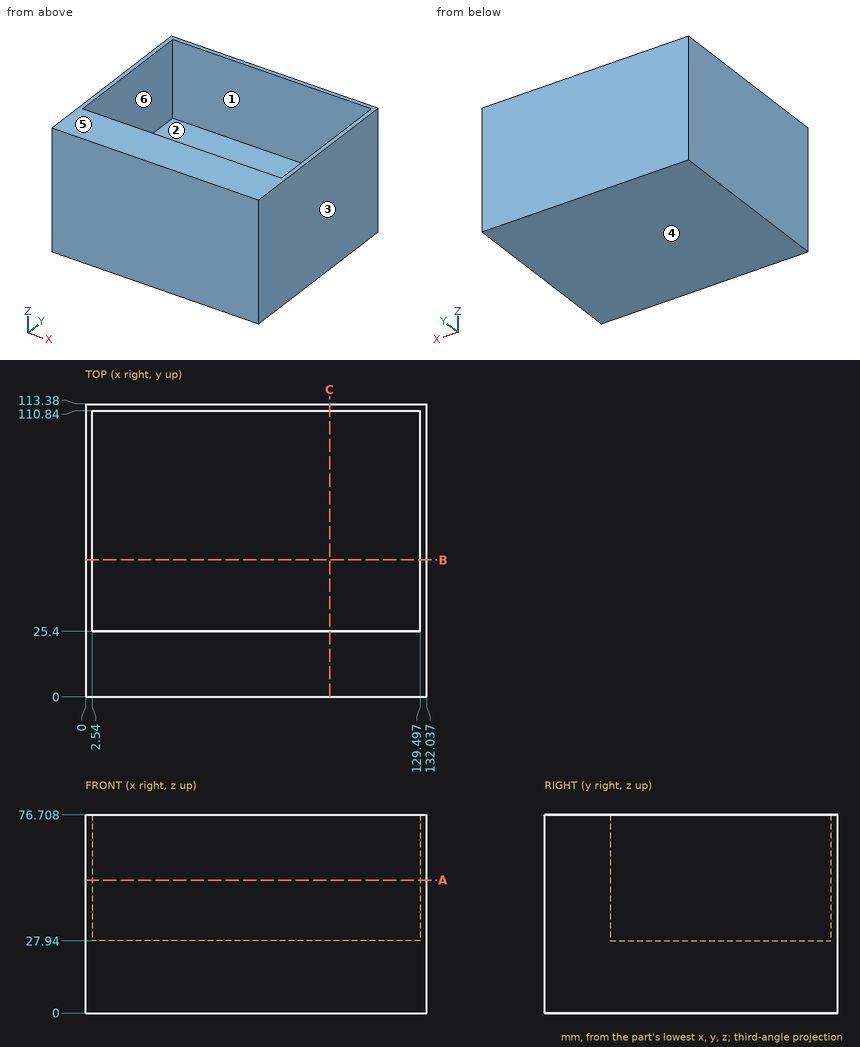
Answer from the drawing. Dimensions are ordinates in mm from the lowest x, y and z of the part. A direction names the side the tool comes from. Give positions to 0.01 mm unless a question says otherwise; leave off trailing zeros. Loops run counter-clockwise (first coordinate to the right, second up) from the corner with the lowest first, then second, coordinate; pieces in that order, holes last. Notation, with made-up numbers: (41.5, 55) - (83.5, 55) arc R38 ccw to (83.5, 94) - close; hole circle Ø5 at (71, -38.75). An arc over 180 degrees is marked (long way). Answer as a JSON object with one key per item and string values.
1. For the marked faces 5 and 6, determine the directions among +Z, -Z, +X, -X, +Y, -Y from which every point of the face is accessible in a straight line to the end or side of a thin tool.
Determined:
{"face 5": "+Z, +X, -X, +Y, -Y", "face 6": "+Z"}
2. For a pull along X with two mould halves and no side action, classify the marked faces 1, 2, 3 and 4 as pulls with the +X half, pulls with the -X half, needs draft (parallel to the pull), parting line crosses it, or undercut.
Determined:
{"face 1": "undercut", "face 2": "undercut", "face 3": "pulls with the +X half", "face 4": "needs draft"}
3. A cutting plane is placed at B-B (y = 53). Write down the section's boundary in (x, z), then the cut area to 3 significant figures.
Determined:
{"outline": "(0, 0) - (132.04, 0) - (132.04, 76.71) - (129.5, 76.71) - (129.5, 27.94) - (2.54, 27.94) - (2.54, 76.71) - (0, 76.71) - close", "area": "3,940 mm²"}
4. Find the intervals of material crossed by L1, parallel to X at y = 104.5, z = 43; L2, parallel to Y at x = 117, z = 72.5; L3, parallel to Z at x = 78, y = 85, in increasing order. Write a range as [from, to].
Determined:
{"L1": "[0, 2.54], [129.5, 132.04]", "L2": "[0, 25.4], [110.84, 113.38]", "L3": "[0, 27.94]"}
5. A cutting plane is placed at A-A (z = 51.5). Write down the section's boundary in (x, y).
Determined:
{"outline": "(0, 0) - (132.04, 0) - (132.04, 113.38) - (0, 113.38) - close; hole (2.54, 25.4) - (129.5, 25.4) - (129.5, 110.84) - (2.54, 110.84) - close"}
6. A cutting plane is placed at C-C (x = 94.5). Write down the section's boundary in (y, z).
Determined:
{"outline": "(0, 0) - (113.38, 0) - (113.38, 76.71) - (110.84, 76.71) - (110.84, 27.94) - (25.4, 27.94) - (25.4, 76.71) - (0, 76.71) - close"}
